Autodesk Inventor part; units mm, degrees
ref_plane "YZ Plane" through (0, 0, 0) normal (1, 0, 0) x (0, 1, 0)
ref_plane "XZ Plane" through (0, 0, 0) normal (0, 1, 0) x (-1, 0, 0)
ref_plane "XY Plane" through (0, 0, 0) normal (0, 0, 1) x (1, 0, 0)
sketch "Sketch1" plane through (0, 0, 0) normal (0, 0, 1) x (1, 0, 0)
  line L0 (0, 0) -> (40, 0)
  line L1 (40, 0) -> (40, 150)
  line L2 (40, 150) -> (0, 150)
  line L3 (0, 150) -> (0, 0)
  circle A0 centre (20, 0) radius 30
  circle A1 centre (20, 150) radius 30
  point P0 (0, 22.3607)
  point P1 (40, 22.3607)
  point P2 (40, 127.6393)
  point P3 (0, 127.6393)
  dimension "d0" = 40
  dimension "d1" = 150
  dimension "d2" = 60
  dimension "d3" = 60
extrude "Extrusion1" add sketch "Sketch1" along normal blind 20
sketch "Sketch2" plane through (0, 0, 20) normal (0, 0, 1) x (1, 0, 0)
  line L0 (10, 0) -> (30, 0)
  line L1 (30, 0) -> (30, -17)
  line L2 (30, -17) -> (10, -17)
  line L3 (10, -17) -> (10, 0)
  line L4 (10, 0) -> (30, 0)
  line L5 (30, 0) -> (30, 36.8)
  line L6 (30, 36.8) -> (10, 36.8)
  line L7 (10, 36.8) -> (10, 0)
  line L8 (10, 36.8) -> (30, 36.8)
  line L9 (30, 36.8) -> (30, 30.8)
  line L10 (30, 30.8) -> (10, 30.8)
  line L11 (10, 30.8) -> (10, 36.8)
  line L12 (10, -17) -> (30, -17)
  line L13 (30, -17) -> (30, -11)
  line L14 (30, -11) -> (10, -11)
  line L15 (10, -11) -> (10, -17)
  line L16 (10, 36.8) -> (30, 36.8)
  line L17 (30, 36.8) -> (30, 33.8)
  line L18 (30, 33.8) -> (10, 33.8)
  line L19 (10, 33.8) -> (10, 36.8)
  line L20 (10, -17) -> (30, -17)
  line L21 (30, -17) -> (30, -14)
  line L22 (30, -14) -> (10, -14)
  line L23 (10, -14) -> (10, -17)
  point P0 (0, 0)
  dimension "d6" = 20
  dimension "d7" = 17
  dimension "d8" = 36.8
  dimension "d9" = 6
  dimension "d10" = 6
  dimension "d11" = 3
extrude "Extrusion2" cut sketch "Sketch2" against normal blind 16 contours L7 L10 L5 L0 | L0 L1 L14 L3
sketch "Sketch3" plane through (0, 0, 0) normal (0, 0, -1) x (-1, 0, 0)
  circle A0 centre (-20, 0) radius 10
  point P0 (0, 0)
  dimension "d14" = 20
extrude "Extrusion3" cut sketch "Sketch3" against normal blind 69.725
sketch "Sketch4" plane through (0, 0, 20) normal (0, 0, 1) x (1, 0, 0)
  line L0 (30, -11) -> (10, -11)
  line L1 (10, -11) -> (10, -17)
  line L2 (10, -17) -> (30, -17)
  line L3 (30, -17) -> (30, -11)
  line L4 (30, 30.8) -> (30, 0)
  line L5 (30, 30.8) -> (10, 30.8)
  line L6 (10, 30.8) -> (10, 36.8)
  line L7 (10, 36.8) -> (30, 36.8)
  line L8 (30, 36.8) -> (30, 30.8)
  line L9 (30, -17) -> (10, -17)
  line L10 (10, -17) -> (10, -14)
  line L11 (10, -14) -> (30, -14)
  line L12 (30, -14) -> (30, -17)
  point P0 (0, 0)
  dimension "d17" = 6
  dimension "d18" = 6
extrude "Extrusion4" cut sketch "Sketch4" against normal blind 6
sketch "Sketch5" plane through (0, 0, 14) normal (0, 0, 1) x (1, 0, 0)
  line L0 (30, 36.8) -> (30, -17)
  line L1 (10, -17) -> (10, 36.8)
  line L2 (30, -17) -> (10, -17)
  line L3 (10, -17) -> (10, -14)
  line L4 (10, -14) -> (30, -14)
  line L5 (30, -14) -> (30, -17)
  line L6 (20, -14) -> (15, -14)
  line L7 (15, -14) -> (15, -13.2117)
  line L8 (15, -13.2117) -> (20, -13.2117)
  line L9 (20, -13.2117) -> (20, -14)
  line L10 (20, -14) -> (25, -14)
  line L11 (25, -14) -> (25, -13.2117)
  line L12 (25, -13.2117) -> (20, -13.2117)
  line L13 (20, -13.2117) -> (20, -14)
  circle A0 centre (25, -14) radius 1.35
  circle A1 centre (15, -14) radius 1.35
  line L14 (10, 36.8) -> (30, 36.8)
  line L15 (10, 30.8) -> (10, 36.8)
  line L16 (30, 36.8) -> (10, 36.8)
  line L17 (10, 36.8) -> (10, 33.8)
  line L18 (10, 33.8) -> (30, 33.8)
  line L19 (30, 33.8) -> (30, 36.8)
  line L20 (20, 33.8) -> (25, 33.8)
  line L21 (25, 33.8) -> (25, 32.7882)
  line L22 (25, 32.7882) -> (20, 32.7882)
  line L23 (20, 32.7882) -> (20, 33.8)
  line L24 (20, 33.8) -> (15, 33.8)
  line L25 (15, 33.8) -> (15, 32.7882)
  line L26 (15, 32.7882) -> (20, 32.7882)
  line L27 (20, 32.7882) -> (20, 33.8)
  circle A2 centre (25, 33.8) radius 1.35
  circle A3 centre (15, 33.8) radius 1.35
  point P0 (0, 0)
  dimension "d21" = 3
  dimension "d22" = 5
  dimension "d23" = 5
  dimension "d24" = 2.7
  dimension "d25" = 2.7
  dimension "d26" = 3
  dimension "d27" = 2.7
  dimension "d28" = 2.7
extrude "Extrusion5" cut sketch "Sketch5" against normal blind 10 contours A2 L22 L21 L18 | L18 A2 | A0 L4 | L4 L11 L12 A0 | L21 L22 A2 L18 | A3 L18 | L18 L25 L26 A3 | L4 A0 L12 L11 | L18 A3 L26 L25 | A1 L8 L7 L4 | L4 A1 | A1 L4 L7 L8
thread "Thread1"
thread "Thread2"
thread "Thread3"
thread "Thread4"
sketch "Sketch6" plane through (0, 0, 0) normal (0, 0, -1) x (-1, 0, 0)
  line L0 (0, 0) -> (-20, 0)
  line L1 (-20, 0) -> (-20, 150)
  line L2 (-20, 150) -> (0, 150)
  line L3 (0, 150) -> (0, 0)
  circle A0 centre (-20, 150) radius 10
  circle A1 centre (-25, 150) radius 1
  circle A2 centre (-15, 150) radius 1
  circle A3 centre (-20, 150) radius 1
  dimension "d39" = 20
  dimension "d40" = 150
  dimension "d41" = 20
  dimension "d42" = 2
  dimension "d43" = 2
  dimension "d44" = 2
extrude "Extrusion6" cut sketch "Sketch6" against normal blind 39.2125 contours A3 L2 L1 | L1 L2 A3 | A2 L2 | L2 A2 | A1
sketch "Sketch7" plane through (0, 0, 20) normal (0, 0, 1) x (1, 0, 0)
  circle A0 centre (20, 150) radius 10
  point P0 (0, 0)
  dimension "d47" = 20
extrude "Extrusion7" cut sketch "Sketch7" against normal blind 16
sketch "Sketch8" plane through (0, 0, 20) normal (0, 0, 1) x (1, 0, 0)
  line L0 (40, 22.3607) -> (40, 127.6393)
  line L1 (0, 127.6393) -> (40, 127.6393)
  line L2 (40, 127.6393) -> (40, 22.3607)
  line L3 (40, 22.3607) -> (0, 22.3607)
  line L4 (0, 22.3607) -> (0, 127.6393)
  line L5 (10, 0) -> (10, 30.8)
  line L6 (10, 22.3607) -> (30, 22.3607)
  line L7 (30, 22.3607) -> (30, 92.3607)
  line L8 (30, 92.3607) -> (10, 92.3607)
  line L9 (10, 92.3607) -> (10, 22.3607)
  line L10 (10, 127.6393) -> (30, 127.6393)
  line L11 (30, 127.6393) -> (30, 57.6393)
  line L12 (30, 57.6393) -> (10, 57.6393)
  line L13 (10, 57.6393) -> (10, 127.6393)
  line L14 (0, 127.6393) -> (10, 92.3607)
  line L15 (30, 92.3607) -> (40, 127.6393)
  line L16 (0, 127.6393) -> (0, 22.3607)
  line L17 (10, 57.6393) -> (0, 22.3607)
  line L18 (30, 57.6393) -> (40, 22.3607)
  point P0 (0, 0)
  dimension "d53" = 20
  dimension "d54" = 70
  dimension "d55" = 70
extrude "Extrusion8" cut sketch "Sketch8" against normal blind 56.675 contours L18 L7 L15 L0 | L17 L4 L14 L9
sketch "Sketch9" plane through (0, 0, 20) normal (0, 0, 1) x (1, 0, 0)
  circle A0 centre (20, 150) radius 10
  circle A1 centre (20, 150) radius 10
  point P0 (0, 0)
extrude "Extrusion9" add sketch "Sketch9" against normal blind 16
sketch "Sketch10" plane through (0, 0, 0) normal (0, 0, -1) x (-1, 0, 0)
  circle A0 centre (-20, 150) radius 1
  circle A1 centre (-20, 150) radius 10
  point P0 (0, 0)
  dimension "d60" = 20
extrude "Extrusion10" cut sketch "Sketch10" against normal blind 16
sketch "Sketch11" plane through (0, 0, 0) normal (0, 0, -1) x (-1, 0, 0)
  circle A0 centre (-20, 150) radius 1
  point P0 (0, 0)
extrude "Extrusion11" add sketch "Sketch11" against normal blind 20
sketch "Sketch12" plane through (20, 150, 0) normal (0, 0, -1) x (-1, 0, 0)
  circle A0 centre (0, 0) radius 1
  point P0 (20, -150)
extrude "Extrusion12" cut sketch "Sketch12" against normal blind 49.85
sketch "Sketch13" plane through (20, 150, 16) normal (0, 0, -1) x (-1, 0, 0)
  circle A0 centre (0, -5) radius 1
  circle A1 centre (0, 5) radius 1
  point P0 (20, -150)
  dimension "d67" = 2
  dimension "d68" = 2
extrude "Extrusion13" cut sketch "Sketch13" against normal blind 42.225
chamfer "Chamfer2" distance 12 angle 45 1 edges at (30, 150, 0)
properties part number "1stArm"
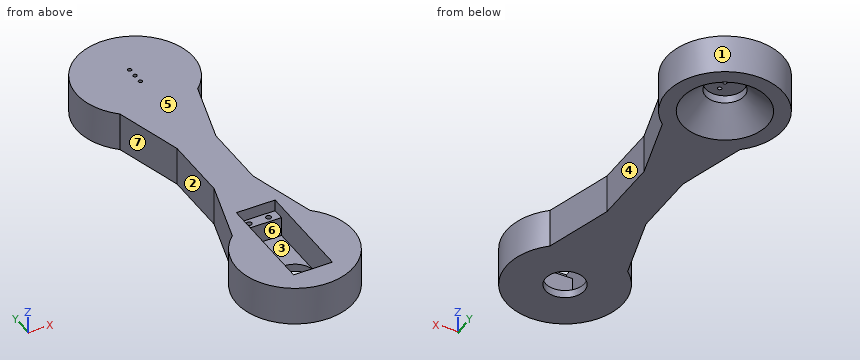
Source: CAD feature listing. Evaluate the final solid. Frame: model axes, mm. Face numbers are marked on the shaded views. A direction names the side the tool comes from. Round coordinates to 2 decimals unless told otherwise and drop trailing zeros. Loops run counter-clockwise (first coordinate to the right, second up) from the corner with the lowest first, then second, coordinate; pieces in that order, holes last. Notation, with made-up numbers: (-23, -27) - (27, -27) arc R15 cw to (27, 2) - close; hole circle Ø11 at (70, -27). An arc over 180 degrees is marked (long way). Write item = value, one per line. Start each with the question number.
(1) Section query B-B, the plane y = -6. Output: boundary loops of the cut face in (x, z).
(2) Ray query, line 1 along Y through (x, z) = (20, 17.3); line 2 along Y through (x, z) = (20, 13.95); line 3 along X through (y, z) = (150, 17). Return the intervals inside material, ascending. Write a range as from..to.
(3) Section query D-D, the plane y = 119. Output: boundary loops of the cut face in (x, z).
(4) Pull-direction query (X, two-part tool) for the marked faces 5, 6 and 7; classes: +X half, -X half, draft (parallel to the pull), parting line (faces both ways), or undercut.
(5) Set-up query: the marked faces 1, 2, 3 and 4. Return all of +Z, -Z, +X, -X, +Y, -Y with unobstructed straight access to the full face (end or side cutting, diameter ignored); none if empty.
(6) Pin query (flat end, axial travel): pin 1 (3 mm diameter, centred on x = 18.5, z = 17, fed in from +Y); pin 2 (5 mm diameter, centred on x = 12.5, z = 15.5, fed in from +Y); pin 3 (1.3 mm diameter, centred on x = 15, y = -14, fed in from +Z). Return the tip coordinate at first contact, or that it passes through.
(7) Section query A-A, the plane x = 44. Output: boundary loops of the cut face in (y, z).
(8) Section query C-C, the plane z = 9.5. State how many separate pieces and enclosed holes the cut face has, plus the area to 3 significant figures.
Conclusion:
q1.outline = (-9.39, 0) - (12, 0) - (12, 4) - (10, 4) - (10, 20) - (-9.39, 20) - close; (28, 0) - (49.39, 0) - (49.39, 20) - (30, 20) - (30, 4) - (28, 4) - close
q2.line_1 = -30..-17, 36.8..144, 146..149, 151..154, 156..180
q2.line_2 = -30..-11, 30.8..140, 160..180
q2.line_3 = -10..19, 21..50
q3.outline = (2.45, 0) - (37.55, 0) - (37.55, 20) - (2.45, 20) - close
q4.face_5 = draft
q4.face_6 = undercut
q4.face_7 = -X half
q5.face_1 = +Z, -Z
q5.face_2 = +Z, -Z, -X
q5.face_3 = +Z
q5.face_4 = +Z, -Z, +X
q6.pin_1 = 180
q6.pin_2 = 179.58
q6.pin_3 = 4
q7.outline = (-18, 0) - (18, 0) - (18, 20) - (-18, 20) - close; (132, 0) - (168, 0) - (168, 20) - (132, 20) - close
q8.separate_pieces = 1
q8.enclosed_holes = 6
q8.area = 6,700 mm2
